Source: CAD feature listing. Evaluate the final solid. Frame: model axes, mm. Face numbers are marked on the shaded views. A direction names the side the tool comes from. Round coordinates to 2 decimals unless told otherwise and drop trailing zeros. Write each loop counter-clockwise with the first axis right and the second up, starting at its lowest first coordinate (ties: lowest second). Pieces come first, ordered by that corner, then holes. Notation, with made-up numbers: M 86,51.5 L 113,51.5 A28 cw 113,83.5 Z; hole C -20,1.5 d8. An arc over 180 degrees is marked long. Answer in a Markdown table with one row per item.
Autodesk Inventor part; units mm, degrees
ref_plane "YZ Plane" through (0, 0, 0) normal (1, 0, 0) x (0, 1, 0)
ref_plane "XZ Plane" through (0, 0, 0) normal (0, 1, 0) x (-1, 0, 0)
ref_plane "XY Plane" through (0, 0, 0) normal (0, 0, 1) x (1, 0, 0)
sketch "Sketch1" plane through (0, 0, 0) normal (0, 1, 0) x (-1, 0, 0)
  line L0 (-15.5, 21.15) -> (15.5, 21.15)
  line L1 (21.15, 15.5) -> (21.15, -15.5)
  line L2 (15.5, -21.15) -> (-15.5, -21.15)
  line L3 (-21.15, -15.5) -> (-21.15, 15.5)
  line L4 (-21.15, 21.15) -> (21.15, -21.15) construction
  line L5 (21.15, 21.15) -> (-21.15, -21.15) construction
  line L6 (-15.5, 15.5) -> (15.5, 15.5)
  line L7 (15.5, 15.5) -> (15.5, -15.5)
  line L8 (15.5, -15.5) -> (-15.5, -15.5)
  line L9 (-15.5, -15.5) -> (-15.5, 15.5)
  line L10 (-15.5, 15.5) -> (15.5, -15.5) construction
  line L11 (15.5, 15.5) -> (-15.5, -15.5) construction
  circle A0 centre (0, 0) radius 11
  circle A1 centre (15.5, 15.5) radius 1.625
  circle A2 centre (15.5, -15.5) radius 1.625
  circle A3 centre (-15.5, -15.5) radius 1.625
  circle A4 centre (-15.5, 15.5) radius 1.625
  line L12 (15.5, -15.5) -> (15.5, -21.15)
  line L13 (21.15, -15.5) -> (15.5, -21.15)
  line L14 (-15.5, -21.15) -> (-21.15, -15.5)
  line L15 (-21.15, 15.5) -> (-15.5, 21.15)
  line L16 (15.5, 21.15) -> (21.15, 15.5)
  line L17 (0, -15.5) -> (0, -21.15)
  line L18 (0, -15.5) -> (0, -18.325)
  line L19 (0, -18.325) -> (0, -21.15)
  circle A5 centre (0, 0) radius 19.7375
  dimension "d0" = 42.3
  dimension "d1" = 42.3
  dimension "d2" = 31
  dimension "d3" = 31
  dimension "d4" = 22
  dimension "d5" = 3.25
  dimension "d6" = 3.25
  dimension "d7" = 3.25
  dimension "d8" = 3.25
extrude "Extrusion1" add sketch "Sketch1" along normal blind 2 contours L0 L16 L1 L13 L12 A2 L7 A5 A1 L6 A4 L9 A3 L8 L17 L2 L14 L3 L15 | L2 L17 A5 L8 A2 L12 | A5 L8 L17 | L17 L8 A5 | L8 A5 L7 A2 | A5 L9 L6 L7 L8 | L8 A3 L9 A5 | A5 L9 | L7 A5 | L9 A4 L6 A5 | A5 L6 A1 L7 | A5 L6
sketch "Sketch2" plane through (0, 2, 0) normal (0, 1, 0) x (1, 0, 0)
  line L0 (-15.5, 21.15) -> (15.5, 21.15)
  line L1 (21.15, 15.5) -> (21.15, -15.5)
  line L2 (15.5, -21.15) -> (-15.5, -21.15)
  line L3 (-21.15, -15.5) -> (-21.15, 15.5)
  line L4 (-21.15, 21.15) -> (21.15, -21.15) construction
  line L5 (21.15, 21.15) -> (-21.15, -21.15) construction
  line L6 (-15.5, 15.5) -> (15.5, 15.5)
  line L7 (15.5, 15.5) -> (15.5, -15.5)
  line L8 (15.5, -15.5) -> (-15.5, -15.5)
  line L9 (-15.5, -15.5) -> (-15.5, 15.5)
  line L10 (-15.5, 15.5) -> (15.5, -15.5) construction
  line L11 (15.5, 15.5) -> (-15.5, -15.5) construction
  circle A0 centre (0, 0) radius 11
  circle A1 centre (15.5, 15.5) radius 1.625
  circle A2 centre (15.5, -15.5) radius 1.625
  circle A3 centre (-15.5, -15.5) radius 1.625
  circle A4 centre (-15.5, 15.5) radius 1.625
  line L12 (15.5, -15.5) -> (15.5, -21.15)
  line L13 (21.15, -15.5) -> (15.5, -21.15)
  line L14 (-15.5, -21.15) -> (-21.15, -15.5)
  line L15 (-21.15, 15.5) -> (-15.5, 21.15)
  line L16 (15.5, 21.15) -> (21.15, 15.5)
  line L17 (0, -15.5) -> (0, -21.15)
  line L18 (0, -15.5) -> (0, -18.325)
  line L19 (0, -18.325) -> (0, -21.15)
  circle A5 centre (0, 0) radius 19.7375
  circle A6 centre (0, 0) radius 11
  line L20 (-15.5, -21.15) -> (15.5, -21.15)
  line L21 (-13.9565, -13.9565) -> (-6.763, -21.15)
  line L22 (0, 0) -> (7.7782, -7.7782) construction
  line L23 (13.9565, 13.9565) -> (21.15, 6.763)
  circle A7 centre (0, 0) radius 14.7375 construction
  line L24 (-1.1373, -19.7047) -> (0.308, -21.15)
  line L25 (19.7047, 1.1373) -> (21.15, -0.308)
  point P0 (-10.421, -10.421)
  point P1 (10.421, 10.421)
  point P2 (20.4274, 0.4146)
  point P3 (15.5, 12.2196)
  point P4 (15.5, 12.413)
  point P5 (-12.413, -15.5)
  point P6 (-12.2196, -15.5)
  point P7 (0, -20.842)
  point P8 (21.15, -0.308)
  dimension "d15" = 22
  dimension "d11" = 42.3
  dimension "d12" = 42.3
  dimension "d13" = 31
  dimension "d14" = 31
  dimension "d16" = 3.25
  dimension "d17" = 3.25
  dimension "d18" = 3.25
  dimension "d19" = 3.25
  dimension "d23" = 5
  dimension "d24" = 5
extrude "Extrusion2" add sketch "Sketch2" along normal blind 6 contours L0 L16 L1 L23 L7 A1 L6 A5 A4 L9 A3 L8 L21 L2 L14 L3 L15 | L1 L13 L12 A2 L7 A5 L25 | L23 A5 L6 A1 L7 | L8 A3 L9 A5 L21 | L2 L24 L17 A5 L8 A2 L12 | L7 A2 L8 A5 | L24 A5 L17 | A5 L9 A4 L6
properties part number "Pumphousing"
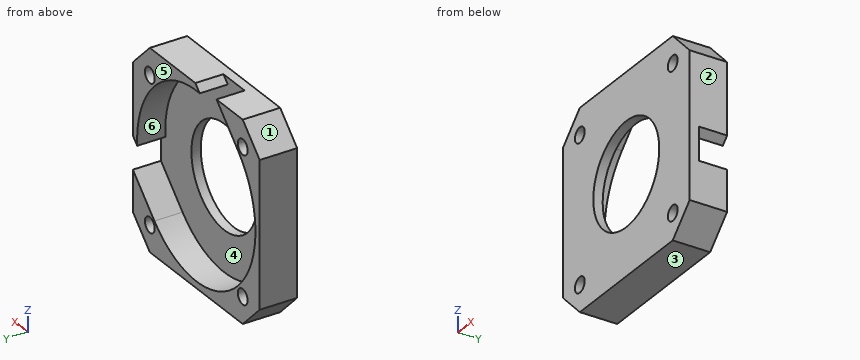
Q1. Access query for the marked faces 5 and 6. Directions: +Z, -Z, +X, -X, +Y, -Y. A direction counts if a zero-diameter tool reaches every point of the face in a straight line with its end or side. Return the directions, or none.
Solutions:
| item | result |
|---|---|
| face 5 | +Z, -Z, +X, -X, +Y |
| face 6 | +Y |
Q2. Section B-B (x = -4). Return loops of the section in (y, z), and give its area (3 significant figures).
Solutions:
| item | result |
|---|---|
| outline | M 0,-21.15 L 8,-21.15 L 8,-19.33 L 2,-19.33 L 2,-10.25 L 0,-10.25 Z; M 0,10.25 L 2,10.25 L 2,21.15 L 0,21.15 Z |
| area | 54.5 mm2 |
Q3. Material intervals for probe 1 along X at (y, z) = (3.5, -15); probe 2 along X at (y, z) = (5.25, 15.5) (3 decimals), sorted ascending.
Solutions:
| item | result |
|---|---|
| probe 1 | x = -21.15 to -17.05, -13.95 to -12.83, 12.83 to 13.95, 17.05 to 21.15 |
| probe 2 | x = -21.15 to -17.125, -13.875 to -12.413, 12.22 to 13.875, 17.125 to 21.15 |
Q4. Section A-A (y = 7.25). State how many separate pieces and enclosed holes the cut face has, and give its area (3 significant figures).
Solutions:
| item | result |
|---|---|
| separate pieces | 2 |
| enclosed holes | 4 |
| area | 432 mm2 |
Q5. Section D-D (z = 11.5). Return loops of the section in (x, y).
Solutions:
| item | result |
|---|---|
| outline | M -21.15,0 L 21.15,0 L 21.15,8 L 16.04,8 L 16.04,2 L -16.04,2 L -16.04,8 L -21.15,8 Z |
Q6. Pull-direction query (X, two-part tool) for the marked faces 1, 2, 3 and 4; classes: pulls with the +X half, pulls with the -X half, needs draft (parallel to the pull), parting line crosses it, or undercut.
Solutions:
| item | result |
|---|---|
| face 1 | pulls with the -X half |
| face 2 | pulls with the +X half |
| face 3 | needs draft |
| face 4 | undercut |
Q7. Section C-C (z = -5). Return loops of the section in (x, y).
Solutions:
| item | result |
|---|---|
| outline | M -21.15,0 L -9.8,0 L -9.8,2 L -19.09,2 L -19.09,8 L -21.15,8 Z; M 9.8,0 L 21.15,0 L 21.15,2 L 9.8,2 Z |
Q8. Contact query for flat-ended pins moving along their axis: pin 1 Ø2.5 at (x, z) = (-15.5, 15.5) entering from +Y; pin 2 Ø12.5 at (x, z) = (9.5, 1) entering from +Y; pin 3 Ø5 at (x, z) = (-13.5, -11) entering from +Y. Output: stop coordinate, or through.
Solutions:
| item | result |
|---|---|
| pin 1 | passes through |
| pin 2 | stops at y = 2 |
| pin 3 | stops at y = 8 |
